Here's how the part is built. I have some questions about the finished solid (model axes, mm). Round coordinates to 2 decimals unless told otherwise and drop trailing zeros. Loops run counter-clockwise (first coordinate to the right, second up) from the corner with the lowest first, then second, coordinate; pieces in that order, holes last. Notation, with made-up numbers: M 78.5,-34 L 98.5,-34 A27 ccw 98.5,-9 Z; hole C 6,-9.75 d5. An arc over 180 degrees is marked long. Answer as a JSON object with one key per item and string values.
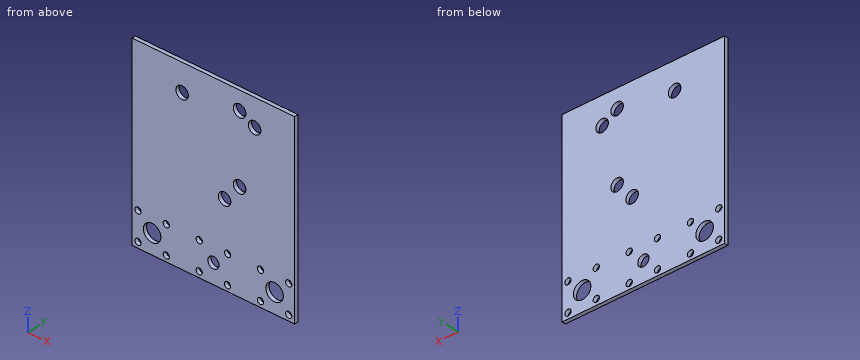
from build123d import *

# Parameters (mm, degrees)
SKETCH1_W                  = 130
SKETCH1_H                  = 150
BOSS_EXTRUDE1_DEPTH        = 3
F_10_0_10_DIAMETER_HOLE2_D = 10
F_14_0_14_DIAMETER_HOLE1_D = 14
F_5_0_5_DIAMETER_HOLE1_D   = 5
F_10_0_10_DIAMETER_HOLE1_D = 10
F_9_0_9_DIAMETER_HOLE1_D   = 9
F_5_0_5_DIAMETER_HOLE2_D   = 5


with BuildPart() as part:
    # Sketch1 → Boss-Extrude1 (new body)
    with BuildSketch(Plane(origin=(0, 0, 0), x_dir=(1, 0, 0), z_dir=(0, 1, 0))):
        with Locations((65, -75)):
            Rectangle(SKETCH1_W, SKETCH1_H)
    extrude(amount=BOSS_EXTRUDE1_DEPTH)

    # Ø10.0 (10) Diameter Hole2 (through all)
    with Locations(Plane(origin=(0, 3, 0), x_dir=(1, 0, 0), z_dir=(0, 1, 0))):
        with Locations((98, -128), (40, -128), (74, -66)):
            Hole(F_10_0_10_DIAMETER_HOLE2_D / 2)

    # Ø14.0 (14) Diameter Hole1 (through all)
    with Locations(Plane(origin=(0, 3, 0), x_dir=(1, 0, 0), z_dir=(0, 1, 0))):
        with Locations((16, -16), (114, -16)):
            Hole(F_14_0_14_DIAMETER_HOLE1_D / 2)

    # Ø5.0 (5) Diameter Hole1 (through all)
    with Locations(Plane(origin=(0, 3, 0), x_dir=(1, 0, 0), z_dir=(0, 1, 0))):
        with Locations((4.686291501, -27.313708499), (4.686291501, -4.686291501), (27.313708499, -4.686291501), (27.313708499, -27.313708499), (102.686291501, -27.313708499), (125.313708499, -27.313708499), (125.313708499, -4.686291501), (102.686291501, -4.686291501)):
            Hole(F_5_0_5_DIAMETER_HOLE1_D / 2)

    # Ø10.0 (10) Diameter Hole1 (through all)
    with Locations(Plane(origin=(0, 3, 0), x_dir=(1, 0, 0), z_dir=(0, 1, 0))):
        with Locations((86, -80), (86, -135)):
            Hole(F_10_0_10_DIAMETER_HOLE1_D / 2)

    # Ø9.0 (9) Diameter Hole1 (through all)
    with Locations(Plane(origin=(0, 3, 0), x_dir=(1, 0, 0), z_dir=(0, 1, 0))):
        with Locations((65, -16)):
            Hole(F_9_0_9_DIAMETER_HOLE1_D / 2)

    # Ø5.0 (5) Diameter Hole2 (through all)
    with Locations(Plane(origin=(0, 3, 0), x_dir=(1, 0, 0), z_dir=(0, 1, 0))):
        with Locations((53.686291501, -27.313708499), (76.313708499, -27.313708499), (76.313708499, -4.686291501), (53.686291501, -4.686291501)):
            Hole(F_5_0_5_DIAMETER_HOLE2_D / 2)


solid = part.part
Item 1: I want a section at C-C, the plane z = 135. Please give me the cut outline in (x, y).
Resolved:
{"outline": "M 0,0 L 81,0 L 81,3 L 0,3 Z; M 91,0 L 130,0 L 130,3 L 91,3 Z"}
Item 2: I want a section at D-D, the plane y = 0.85. State how many separate pieces and enclosed holes the cut face has, then the cut area to 3 significant figures.
Resolved:
{"separate pieces": "1", "enclosed holes": "20", "area": "18,500 mm²"}
Item 3: I want a section at B-B, the plane x = 40. Please give me the cut outline in (y, z), then the cut area to 3 significant figures.
Resolved:
{"outline": "M 0,0 L 3,0 L 3,123 L 0,123 Z; M 0,133 L 3,133 L 3,150 L 0,150 Z", "area": "420 mm²"}
Item 4: Please list where these lines run through material, in increasing order: probe 1 along X at (y, z) = (2, 16); probe 2 along X at (y, z) = (1.7, 128); probe 3 along Z at (x, y) = (86, 0.9). Write a range as from..to.
Resolved:
{"probe 1": "0..9, 23..60.5, 69.5..107, 121..130", "probe 2": "0..35, 45..93, 103..130", "probe 3": "0..75, 85..130, 140..150"}
Item 5: I want a section at A-A, the plane z = 16. Please give me the cut outline in (x, y).
Resolved:
{"outline": "M 0,0 L 9,0 L 9,3 L 0,3 Z; M 23,0 L 60.5,0 L 60.5,3 L 23,3 Z; M 69.5,0 L 107,0 L 107,3 L 69.5,3 Z; M 121,0 L 130,0 L 130,3 L 121,3 Z"}
